```python
from build123d import *

# Parameters (mm, degrees)
SKETCH1_W           = 55
SKETCH1_H           = 80
SKETCH1_R           = 13
SKETCH1_R_2         = 2.15
BOSS_EXTRUDE2_DEPTH = 3
SKETCH2_W           = 55
SKETCH2_H           = 3
BOSS_EXTRUDE3_DEPTH = 80
SKETCH3_W           = 3
SKETCH3_H           = 10
CUT_EXTRUDE1_DEPTH  = 80
SKETCH4_W           = 55
SKETCH4_H           = 25
BOSS_EXTRUDE4_DEPTH = 3
SKETCH5_W           = 55
SKETCH5_H           = 3
CUT_EXTRUDE2_DEPTH  = 22
BOSS_EXTRUDE5_DEPTH = 3
BOSS_EXTRUDE6_DEPTH = 3


with BuildPart() as part:
    # Sketch1 → Boss-Extrude2 (new body)
    with BuildSketch(Plane(origin=(0, 0, 0), x_dir=(1, 0, 0), z_dir=(0, 1, 0))):
        Rectangle(SKETCH1_W, SKETCH1_H)
        with Locations((0, -12.743931666)):
            Circle(SKETCH1_R, mode=Mode.SUBTRACT)
        with Locations((12.374368671, -0.369562995)):
            Circle(SKETCH1_R_2, mode=Mode.SUBTRACT)
        with Locations((12.374368671, -25.118300337)):
            Circle(SKETCH1_R_2, mode=Mode.SUBTRACT)
        with Locations((-12.374368671, -25.118300337)):
            Circle(SKETCH1_R_2, mode=Mode.SUBTRACT)
        with Locations((-12.374368671, -0.369562995)):
            Circle(SKETCH1_R_2, mode=Mode.SUBTRACT)
    extrude(amount=BOSS_EXTRUDE2_DEPTH)

    # Sketch2 → Boss-Extrude3 (add)
    with BuildSketch(Plane.XZ):
        with Locations((0, -13.5)):
            Rectangle(SKETCH2_W, SKETCH2_H)
    extrude(amount=BOSS_EXTRUDE3_DEPTH)

    # Sketch3 → Cut-Extrude1 (cut)
    with BuildSketch(Plane(origin=(0, 0, -15), x_dir=(-1, 0, 0), z_dir=(0, 0, -1))):
        with Locations((0, -60)):
            Rectangle(SKETCH3_W, SKETCH3_H)
    extrude(amount=-CUT_EXTRUDE1_DEPTH, mode=Mode.SUBTRACT)

    # Sketch4 → Boss-Extrude4 (add)
    with BuildSketch(Plane(origin=(0, 0, -40), x_dir=(-1, 0, 0), z_dir=(0, 0, -1))):
        with Locations((0, -9.5)):
            Rectangle(SKETCH4_W, SKETCH4_H)
    extrude(amount=BOSS_EXTRUDE4_DEPTH)

    # Sketch5 → Cut-Extrude2 (cut)
    with BuildSketch(Plane.XZ.offset(22)):
        with Locations((0, -41.5)):
            Rectangle(SKETCH5_W, SKETCH5_H)
    extrude(amount=-CUT_EXTRUDE2_DEPTH, mode=Mode.SUBTRACT)

    # Sketch6 → Boss-Extrude5 (add)
    with BuildSketch(Plane(origin=(27.5, 0, 0), x_dir=(0, 0, -1), z_dir=(1, 0, 0))):
        Polygon((-40, 0), (12, 0), (12, -52), align=None)
    extrude(amount=-BOSS_EXTRUDE5_DEPTH)

    # Sketch7 → Boss-Extrude6 (add)
    with BuildSketch(Plane.ZY.offset(27.5)):
        Polygon((-12, 0), (40, 0), (-12, -52), align=None)
    extrude(amount=-BOSS_EXTRUDE6_DEPTH)


solid = part.part
```
Part model, mm, in its own coordinate system. A direction names the side the tool comes from. Coordinates: 2 decimals unless noted, no trailing zeros. Write each loop counter-clockwise with the first axis right and the second up, starting at its lowest first coordinate (ties: lowest second). Pieces come first, ordered by that corner, then holes.
Item 1: Which spindle directions (+Z, -Z, +X, -X, +Y, -Y) get a long thin tool onto all of the face, cutting with end or side? Do faces 5 (the face through (24.5, -20, 8)), 6 (the face through (1.5, -60, -14)), 7 (the face through (0, 0, -29)), 8 (the face through (-12.84, 1.479, 27.217)), 9 (the face through (27.5, -20, 1)). Say none if no direction does.
Item 2: Slice it at D-D (x = 17). Write the cut outline in (y, z).
Item 3: Probe line 1 (Z direction, x = 0, y = 1); line 2 (X direction, y = -22, z = -3); line 3 (Y direction, x = -7.5, z = -2.5). List the from-to ranges inside material, lowest first.
Item 4: Mould opens along Y. For faces 1 (the face through (0, 2, -43)), 2 (the face through (0, -65, -14)), 3 (the face through (0, 3, -1)), 4 (the face through (-1.5, -60, -14)) say: released by +Y, released by -Y, zero draft, split by the parting line, or undercut.
Item 5: Slice it at B-B (y = -60.5). Write the cut outline in (x, z).
Item 6: Pin check, flat tips, straight feed: pin 1 (7 mm diameter, centred on x = -12.37, z = 0.37, fed in from -Y); pin 2 (1 mm diameter, centred on x = 7.5, y = -49.5, fed in from -Z); pin 3 (10 mm diameter, centred on x = -3.5, y = -28, fed in from +Z). Stop position of each tip, or through.
Item 7: Slice it at A-A (x = 0). Write the cut outline in (y, z).
Item 8: Slice it at C-C (y = -23.5). Write the cut outline in (x, z).
Results found:
1. face 5: +Z, -Y
1. face 6: +Z, -Z
1. face 7: -Z, +X, -X, -Y
1. face 8: +Y, -Y
1. face 9: +Z, -Z, +X, +Y, -Y
2. outline: (-80, -15) - (0, -15) - (0, -43) - (3, -43) - (3, 40) - (0, 40) - (0, -12) - (-80, -12) - close
3. line 1: z = -43 to -0.26, 25.74 to 40
3. line 2: x = -27.5 to -24.5, 24.5 to 27.5
3. line 3: y = 0 to 3
4. face 1: zero draft
4. face 2: undercut
4. face 3: released by +Y
4. face 4: undercut
5. outline: (-27.5, -15) - (-1.5, -15) - (-1.5, -12) - (-27.5, -12) - close; (1.5, -15) - (27.5, -15) - (27.5, -12) - (1.5, -12) - close
6. pin 1: stops at y = 0
6. pin 2: stops at z = -15
6. pin 3: stops at z = -12
7. outline: (-80, -15) - (-65, -15) - (-65, -12) - (-80, -12) - close; (-55, -15) - (0, -15) - (0, -43) - (3, -43) - (3, -0.26) - (0, -0.26) - (0, -12) - (-55, -12) - close; (0, 25.74) - (3, 25.74) - (3, 40) - (0, 40) - close
8. outline: (-27.5, -15) - (27.5, -15) - (27.5, 16.5) - (24.5, 16.5) - (24.5, -12) - (-24.5, -12) - (-24.5, 16.5) - (-27.5, 16.5) - close
